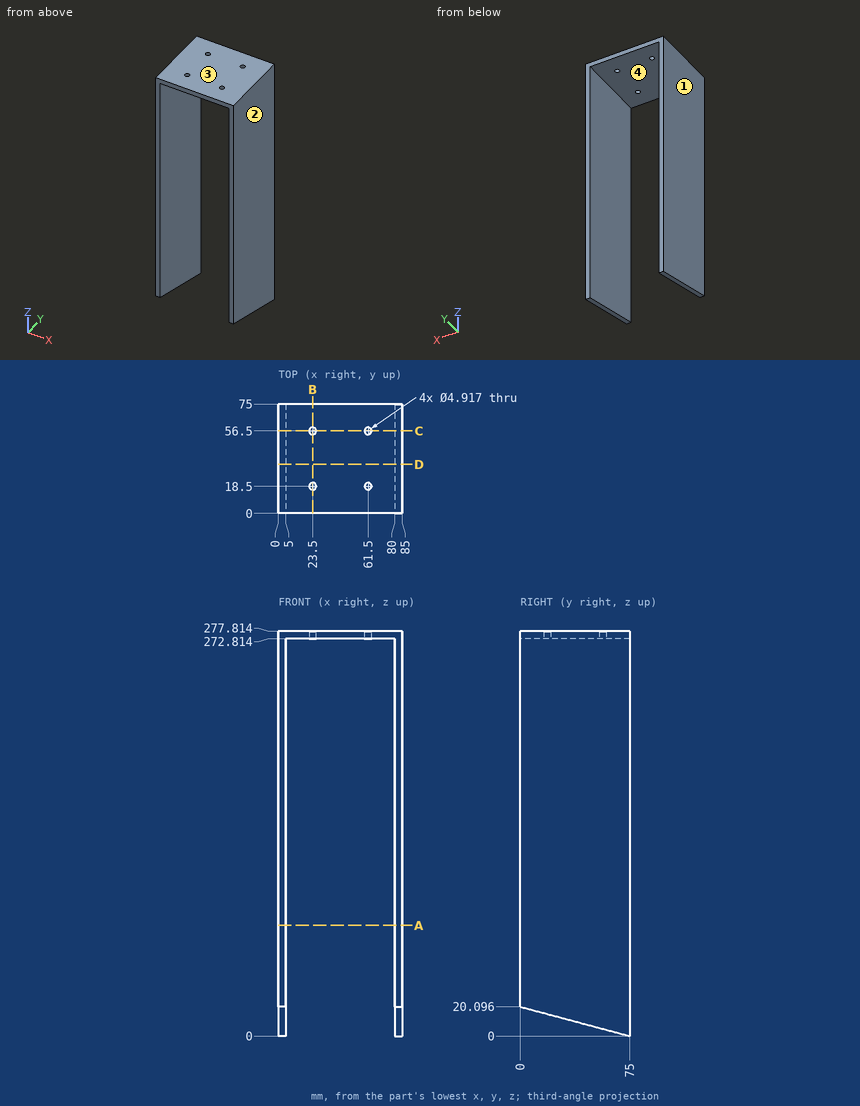
The figure shows three views and two pictorial views of one solid part (mm, origin at its lowest corner). Answer the questions. Round coordinates to 2 decimals unless told otherwise and drop trailing zeros. Order: outer loops, then holes, each group sorted by start corner. A loop starts at its lowest first (then second) coordinate and runs counter-clockwise, first axis right, second up.
Q1. A cutting plane is placed at A-A, the plane z = 76. Determine the outline of the cut face in (x, y).
Solution:
outline: (0, 0) - (5, 0) - (5, 75) - (0, 75) - close; (80, 0) - (85, 0) - (85, 75) - (80, 75) - close
Q2. Find the intervals of material crossed by line 1 along Y through (x, z) = (61, 273); line 2 along Y through (x, z) = (23.5, 274.15); line 3 along X through (y, z) = (3.5, 67), in increasing order.
Solution:
line 1: y = 0 to 16.09, 20.91 to 54.09, 58.91 to 75
line 2: y = 0 to 16.04, 20.96 to 54.04, 58.96 to 75
line 3: x = 0 to 5, 80 to 85
Q3. The mould has two halves that part along X. Classify the marked faces 1, 2, 3 and 4: pulls with the +X half, pulls with the -X half, needs draft (parallel to the pull), parting line crosses it, or undercut.
Solution:
face 1: pulls with the -X half
face 2: pulls with the +X half
face 3: needs draft
face 4: undercut
Q4. A cutting plane is placed at D-D, the plane y = 33.5. Determine the outline of the cut face in (x, z), then the cut area to 3 significant figures.
Solution:
outline: (0, 11.12) - (5, 11.12) - (5, 272.81) - (80, 272.81) - (80, 11.12) - (85, 11.12) - (85, 277.81) - (0, 277.81) - close
area: 3,040 mm2
Q5. A cutting plane is placed at B-B, the plane x = 23.5. Determine the outline of the cut face in (y, z).
Solution:
outline: (0, 272.81) - (16.04, 272.81) - (16.04, 277.81) - (0, 277.81) - close; (20.96, 272.81) - (54.04, 272.81) - (54.04, 277.81) - (20.96, 277.81) - close; (58.96, 272.81) - (75, 272.81) - (75, 277.81) - (58.96, 277.81) - close
Q6. A cutting plane is placed at C-C, the plane y = 56.5. Determine the outline of the cut face in (x, z).
Solution:
outline: (0, 4.96) - (5, 4.96) - (5, 272.81) - (21.04, 272.81) - (21.04, 277.81) - (0, 277.81) - close; (25.96, 272.81) - (59.04, 272.81) - (59.04, 277.81) - (25.96, 277.81) - close; (63.96, 272.81) - (80, 272.81) - (80, 4.96) - (85, 4.96) - (85, 277.81) - (63.96, 277.81) - close
Q7. Given pin 1 Ø4.5 at (x, y) = (23.5, 56.5) entering from -Z; pin 2 Ø3 at (y, z) = (12, 148) entering from -X; pin 3 Ø1.5 at (x, y) = (48, 59) entering from -Z, each flat-ended and moving along its own axis, determine where each tip first touches the part or whether it passes through.
Solution:
pin 1: passes through
pin 2: stops at x = 0
pin 3: stops at z = 272.81
